```python
from build123d import *

# Parameters (mm, degrees)
SKETCH2_W                 = 130
SKETCH2_H                 = 130
BOSS_EXTRUDE1_DEPTH       = 3.2
CUT_EXTRUDE1_REACH        = 93.98
SKETCH4_R                 = 1.7
CUT_EXTRUDE2_REACH        = 93.98
SKETCH6_R                 = 1.7
CUT_EXTRUDE3_REACH        = 93.98
SKETCH8_R                 = 1.7
PRIMARY_WIRE_HOLE_REACH   = 93.98
SKETCH9_R                 = 2.25
SECONDARY_WIRE_HOLE_REACH = 93.98
SKETCH10_R                = 1.25
CUT_EXTRUDE6_REACH        = 93.98


with BuildPart() as part:
    # Sketch2 → Boss-Extrude1 (new body)
    with BuildSketch(Plane(origin=(0, 0, 0), x_dir=(1, 0, 0), z_dir=(0, 1, 0))):
        Rectangle(SKETCH2_W, SKETCH2_H)
    extrude(amount=BOSS_EXTRUDE1_DEPTH)

    # Sketch4 → Cut-Extrude1 (cut, up to next)
    with BuildSketch(Plane(origin=(0, 3.2, 0), x_dir=(1, 0, 0), z_dir=(0, 1, 0)), mode=Mode.PRIVATE) as cut_extrude1_sk1:
        with Locations(Location((-57.3, 57.3, 0), (0, 0, 270))):
            Circle(SKETCH4_R)
    cut_extrude1_tool1 = extrude(cut_extrude1_sk1.sketch, amount=-CUT_EXTRUDE1_REACH, mode=Mode.PRIVATE) & part.part
    # Sketch4 → Cut-Extrude1 (cut, up to next)
    with BuildSketch(Plane(origin=(0, 3.2, 0), x_dir=(1, 0, 0), z_dir=(0, 1, 0)), mode=Mode.PRIVATE) as cut_extrude1_sk2:
        with Locations(Location((57.3, 57.3, 0), (0, 0, 270))):
            Circle(SKETCH4_R)
    cut_extrude1_tool2 = extrude(cut_extrude1_sk2.sketch, amount=-CUT_EXTRUDE1_REACH, mode=Mode.PRIVATE) & part.part
    # Sketch4 → Cut-Extrude1 (cut, up to next)
    with BuildSketch(Plane(origin=(0, 3.2, 0), x_dir=(1, 0, 0), z_dir=(0, 1, 0)), mode=Mode.PRIVATE) as cut_extrude1_sk3:
        with Locations(Location((57.3, -57.3, 0), (0, 0, 270))):
            Circle(SKETCH4_R)
    cut_extrude1_tool3 = extrude(cut_extrude1_sk3.sketch, amount=-CUT_EXTRUDE1_REACH, mode=Mode.PRIVATE) & part.part
    # Sketch4 → Cut-Extrude1 (cut, up to next)
    with BuildSketch(Plane(origin=(0, 3.2, 0), x_dir=(1, 0, 0), z_dir=(0, 1, 0)), mode=Mode.PRIVATE) as cut_extrude1_sk4:
        with Locations(Location((-57.3, -57.3, 0), (0, 0, 270))):
            Circle(SKETCH4_R)
    cut_extrude1_tool4 = extrude(cut_extrude1_sk4.sketch, amount=-CUT_EXTRUDE1_REACH, mode=Mode.PRIVATE) & part.part
    add(cut_extrude1_tool1.solids().sort_by_distance((-57.3, 3.2, -57.3))[0], mode=Mode.SUBTRACT)
    add(cut_extrude1_tool2.solids().sort_by_distance((57.3, 3.2, -57.3))[0], mode=Mode.SUBTRACT)
    add(cut_extrude1_tool3.solids().sort_by_distance((57.3, 3.2, 57.3))[0], mode=Mode.SUBTRACT)
    add(cut_extrude1_tool4.solids().sort_by_distance((-57.3, 3.2, 57.3))[0], mode=Mode.SUBTRACT)

    # Sketch6 → Cut-Extrude2 (cut, up to next)
    with BuildSketch(Plane(origin=(0, 3.2, 0), x_dir=(1, 0, 0), z_dir=(0, 1, 0)), mode=Mode.PRIVATE) as cut_extrude2_sk1:
        with Locations(Location((-40.305086528, 40.305086528, 0), (0, 0, 270))):
            Circle(SKETCH6_R)
    cut_extrude2_tool1 = extrude(cut_extrude2_sk1.sketch, amount=-CUT_EXTRUDE2_REACH, mode=Mode.PRIVATE) & part.part
    # Sketch6 → Cut-Extrude2 (cut, up to next)
    with BuildSketch(Plane(origin=(0, 3.2, 0), x_dir=(1, 0, 0), z_dir=(0, 1, 0)), mode=Mode.PRIVATE) as cut_extrude2_sk2:
        with Locations(Location((40.305086528, 40.305086528, 0), (0, 0, 270))):
            Circle(SKETCH6_R)
    cut_extrude2_tool2 = extrude(cut_extrude2_sk2.sketch, amount=-CUT_EXTRUDE2_REACH, mode=Mode.PRIVATE) & part.part
    # Sketch6 → Cut-Extrude2 (cut, up to next)
    with BuildSketch(Plane(origin=(0, 3.2, 0), x_dir=(1, 0, 0), z_dir=(0, 1, 0)), mode=Mode.PRIVATE) as cut_extrude2_sk3:
        with Locations(Location((40.305086528, -40.305086528, 0), (0, 0, 270))):
            Circle(SKETCH6_R)
    cut_extrude2_tool3 = extrude(cut_extrude2_sk3.sketch, amount=-CUT_EXTRUDE2_REACH, mode=Mode.PRIVATE) & part.part
    # Sketch6 → Cut-Extrude2 (cut, up to next)
    with BuildSketch(Plane(origin=(0, 3.2, 0), x_dir=(1, 0, 0), z_dir=(0, 1, 0)), mode=Mode.PRIVATE) as cut_extrude2_sk4:
        with Locations(Location((-40.305086528, -40.305086528, 0), (0, 0, 270))):
            Circle(SKETCH6_R)
    cut_extrude2_tool4 = extrude(cut_extrude2_sk4.sketch, amount=-CUT_EXTRUDE2_REACH, mode=Mode.PRIVATE) & part.part
    add(cut_extrude2_tool1.solids().sort_by_distance((-40.305087, 3.2, -40.305087))[0], mode=Mode.SUBTRACT)
    add(cut_extrude2_tool2.solids().sort_by_distance((40.305087, 3.2, -40.305087))[0], mode=Mode.SUBTRACT)
    add(cut_extrude2_tool3.solids().sort_by_distance((40.305087, 3.2, 40.305087))[0], mode=Mode.SUBTRACT)
    add(cut_extrude2_tool4.solids().sort_by_distance((-40.305087, 3.2, 40.305087))[0], mode=Mode.SUBTRACT)

    # Sketch8 → Cut-Extrude3 (cut, up to next)
    with BuildSketch(Plane(origin=(0, 3.2, 0), x_dir=(1, 0, 0), z_dir=(0, 1, 0)), mode=Mode.PRIVATE) as cut_extrude3_sk1:
        with Locations(Location((0, 9.5, 0), (0, 0, 270))):
            Circle(SKETCH8_R)
    cut_extrude3_tool1 = extrude(cut_extrude3_sk1.sketch, amount=-CUT_EXTRUDE3_REACH, mode=Mode.PRIVATE) & part.part
    # Sketch8 → Cut-Extrude3 (cut, up to next)
    with BuildSketch(Plane(origin=(0, 3.2, 0), x_dir=(1, 0, 0), z_dir=(0, 1, 0)), mode=Mode.PRIVATE) as cut_extrude3_sk2:
        with Locations(Location((8.227241336, -4.75, 0), (0, 0, 270))):
            Circle(SKETCH8_R)
    cut_extrude3_tool2 = extrude(cut_extrude3_sk2.sketch, amount=-CUT_EXTRUDE3_REACH, mode=Mode.PRIVATE) & part.part
    # Sketch8 → Cut-Extrude3 (cut, up to next)
    with BuildSketch(Plane(origin=(0, 3.2, 0), x_dir=(1, 0, 0), z_dir=(0, 1, 0)), mode=Mode.PRIVATE) as cut_extrude3_sk3:
        with Locations(Location((-8.227241336, -4.75, 0), (0, 0, 270))):
            Circle(SKETCH8_R)
    cut_extrude3_tool3 = extrude(cut_extrude3_sk3.sketch, amount=-CUT_EXTRUDE3_REACH, mode=Mode.PRIVATE) & part.part
    add(cut_extrude3_tool1.solids().sort_by_distance((0, 3.2, -9.5))[0], mode=Mode.SUBTRACT)
    add(cut_extrude3_tool2.solids().sort_by_distance((8.227241, 3.2, 4.75))[0], mode=Mode.SUBTRACT)
    add(cut_extrude3_tool3.solids().sort_by_distance((-8.227241, 3.2, 4.75))[0], mode=Mode.SUBTRACT)

    # Sketch9 → Primary wire hole (cut, up to next)
    with BuildSketch(Plane(origin=(0, 3.2, 0), x_dir=(1, 0, 0), z_dir=(0, 1, 0)), mode=Mode.PRIVATE) as primary_wire_hole_sk1:
        with Locations(Location((48.790367902, 48.790367902, 0), (0, 0, 270))):
            Circle(SKETCH9_R)
    primary_wire_hole_tool1 = extrude(primary_wire_hole_sk1.sketch, amount=-PRIMARY_WIRE_HOLE_REACH, mode=Mode.PRIVATE) & part.part
    add(primary_wire_hole_tool1.solids().sort_by_distance((48.790368, 3.2, -48.790368))[0], mode=Mode.SUBTRACT)

    # Sketch10 → Secondary wire hole (cut, up to next)
    with BuildSketch(Plane(origin=(0, 3.2, 0), x_dir=(1, 0, 0), z_dir=(0, 1, 0)), mode=Mode.PRIVATE) as secondary_wire_hole_sk1:
        with Locations(Location((22.506385739, 18.885099973, 0), (0, 0, 270))):
            Circle(SKETCH10_R)
    secondary_wire_hole_tool1 = extrude(secondary_wire_hole_sk1.sketch, amount=-SECONDARY_WIRE_HOLE_REACH, mode=Mode.PRIVATE) & part.part
    add(secondary_wire_hole_tool1.solids().sort_by_distance((22.506386, 3.2, -18.8851))[0], mode=Mode.SUBTRACT)

    # Sketch11 → Cut-Extrude6 (cut, up to next)
    with BuildSketch(Plane(origin=(0, 3.2, 0), x_dir=(1, 0, 0), z_dir=(0, 1, 0)), mode=Mode.PRIVATE) as cut_extrude6_sk1:
        with BuildLine():
            Line((-34.259927979, 48.372330261), (-15.380990703, 23.319134311))
            ThreePointArc((-15.380990703, 23.319134311), (-15.725426555, 20.868345878), (-18.176214988, 21.21278173))
            Line((-18.176214988, 21.21278173), (-37.055152264, 46.26597768))
            ThreePointArc((-37.055152264, 46.26597768), (-36.710716412, 48.716766113), (-34.259927979, 48.372330261))
        make_face()
    cut_extrude6_tool1 = extrude(cut_extrude6_sk1.sketch, amount=-CUT_EXTRUDE6_REACH, mode=Mode.PRIVATE) & part.part
    # Sketch11 → Cut-Extrude6 (cut, up to next)
    with BuildSketch(Plane(origin=(0, 3.2, 0), x_dir=(1, 0, 0), z_dir=(0, 1, 0)), mode=Mode.PRIVATE) as cut_extrude6_sk2:
        with BuildLine():
            Line((-27.938203096, 52.278884913), (-13.975987518, 24.187365977))
            ThreePointArc((-13.975987518, 24.187365977), (-11.629987027, 23.399151731), (-10.841772782, 25.745152222))
            Line((-10.841772782, 25.745152222), (-24.80398836, 53.836671159))
            ThreePointArc((-24.80398836, 53.836671159), (-27.149988851, 54.624885404), (-27.938203096, 52.278884913))
        make_face()
    cut_extrude6_tool2 = extrude(cut_extrude6_sk2.sketch, amount=-CUT_EXTRUDE6_REACH, mode=Mode.PRIVATE) & part.part
    # Sketch11 → Cut-Extrude6 (cut, up to next)
    with BuildSketch(Plane(origin=(0, 3.2, 0), x_dir=(1, 0, 0), z_dir=(0, 1, 0)), mode=Mode.PRIVATE) as cut_extrude6_sk3:
        with BuildLine():
            Line((-17.87286129, 56.517128637), (-9.301329978, 26.340883824))
            ThreePointArc((-9.301329978, 26.340883824), (-7.139754963, 25.135647974), (-5.934519112, 27.297222989))
            Line((-5.934519112, 27.297222989), (-14.506050425, 57.473467801))
            ThreePointArc((-14.506050425, 57.473467801), (-16.667625439, 58.678703651), (-17.87286129, 56.517128637))
        make_face()
    cut_extrude6_tool3 = extrude(cut_extrude6_sk3.sketch, amount=-CUT_EXTRUDE6_REACH, mode=Mode.PRIVATE) & part.part
    # Sketch11 → Cut-Extrude6 (cut, up to next)
    with BuildSketch(Plane(origin=(0, 3.2, 0), x_dir=(1, 0, 0), z_dir=(0, 1, 0)), mode=Mode.PRIVATE) as cut_extrude6_sk4:
        with BuildLine():
            Line((-7.200805802, 58.836837065), (-4.310928692, 27.600231771))
            ThreePointArc((-4.310928692, 27.600231771), (-2.407156164, 26.018887355), (-0.825811748, 27.922659883))
            Line((-0.825811748, 27.922659883), (-3.715688858, 59.159265177))
            ThreePointArc((-3.715688858, 59.159265177), (-5.619461386, 60.740609593), (-7.200805802, 58.836837065))
        make_face()
    cut_extrude6_tool4 = extrude(cut_extrude6_sk4.sketch, amount=-CUT_EXTRUDE6_REACH, mode=Mode.PRIVATE) & part.part
    # Sketch11 → Cut-Extrude6 (cut, up to next)
    with BuildSketch(Plane(origin=(0, 3.2, 0), x_dir=(1, 0, 0), z_dir=(0, 1, 0)), mode=Mode.PRIVATE) as cut_extrude6_sk5:
        with BuildLine():
            Line((3.715688858, 59.159265177), (0.825811748, 27.922659883))
            ThreePointArc((0.825811748, 27.922659883), (2.407156164, 26.018887355), (4.310928692, 27.600231771))
            Line((4.310928692, 27.600231771), (7.200805802, 58.836837065))
            ThreePointArc((7.200805802, 58.836837065), (5.619461386, 60.740609593), (3.715688858, 59.159265177))
        make_face()
    cut_extrude6_tool5 = extrude(cut_extrude6_sk5.sketch, amount=-CUT_EXTRUDE6_REACH, mode=Mode.PRIVATE) & part.part
    # Sketch11 → Cut-Extrude6 (cut, up to next)
    with BuildSketch(Plane(origin=(0, 3.2, 0), x_dir=(1, 0, 0), z_dir=(0, 1, 0)), mode=Mode.PRIVATE) as cut_extrude6_sk6:
        with BuildLine():
            Line((14.506050425, 57.473467801), (5.934519112, 27.297222989))
            ThreePointArc((5.934519112, 27.297222989), (7.139754963, 25.135647974), (9.301329978, 26.340883824))
            Line((9.301329978, 26.340883824), (17.87286129, 56.517128637))
            ThreePointArc((17.87286129, 56.517128637), (16.667625439, 58.678703651), (14.506050425, 57.473467801))
        make_face()
    cut_extrude6_tool6 = extrude(cut_extrude6_sk6.sketch, amount=-CUT_EXTRUDE6_REACH, mode=Mode.PRIVATE) & part.part
    # Sketch11 → Cut-Extrude6 (cut, up to next)
    with BuildSketch(Plane(origin=(0, 3.2, 0), x_dir=(1, 0, 0), z_dir=(0, 1, 0)), mode=Mode.PRIVATE) as cut_extrude6_sk7:
        with BuildLine():
            Line((24.80398836, 53.836671159), (10.841772782, 25.745152222))
            ThreePointArc((10.841772782, 25.745152222), (11.629987027, 23.399151731), (13.975987518, 24.187365977))
            Line((13.975987518, 24.187365977), (27.938203096, 52.278884913))
            ThreePointArc((27.938203096, 52.278884913), (27.149988851, 54.624885404), (24.80398836, 53.836671159))
        make_face()
    cut_extrude6_tool7 = extrude(cut_extrude6_sk7.sketch, amount=-CUT_EXTRUDE6_REACH, mode=Mode.PRIVATE) & part.part
    # Sketch11 → Cut-Extrude6 (cut, up to next)
    with BuildSketch(Plane(origin=(0, 3.2, 0), x_dir=(1, 0, 0), z_dir=(0, 1, 0)), mode=Mode.PRIVATE) as cut_extrude6_sk8:
        with BuildLine():
            Line((34.259927979, 48.372330261), (15.380990703, 23.319134311))
            ThreePointArc((15.380990703, 23.319134311), (15.725426555, 20.868345878), (18.176214988, 21.21278173))
            Line((18.176214988, 21.21278173), (37.055152264, 46.26597768))
            ThreePointArc((37.055152264, 46.26597768), (36.710716412, 48.716766113), (34.259927979, 48.372330261))
        make_face()
    cut_extrude6_tool8 = extrude(cut_extrude6_sk8.sketch, amount=-CUT_EXTRUDE6_REACH, mode=Mode.PRIVATE) & part.part
    add(cut_extrude6_tool1.solids().sort_by_distance((-26.218071, 3.2, -34.792556))[0], mode=Mode.SUBTRACT)
    add(cut_extrude6_tool2.solids().sort_by_distance((-19.389988, 3.2, -39.012019))[0], mode=Mode.SUBTRACT)
    add(cut_extrude6_tool3.solids().sort_by_distance((-11.90369, 3.2, -41.907176))[0], mode=Mode.SUBTRACT)
    add(cut_extrude6_tool4.solids().sort_by_distance((-4.013309, 3.2, -43.379748))[0], mode=Mode.SUBTRACT)
    add(cut_extrude6_tool5.solids().sort_by_distance((4.013309, 3.2, -43.379748))[0], mode=Mode.SUBTRACT)
    add(cut_extrude6_tool6.solids().sort_by_distance((11.90369, 3.2, -41.907176))[0], mode=Mode.SUBTRACT)
    add(cut_extrude6_tool7.solids().sort_by_distance((19.389988, 3.2, -39.012019))[0], mode=Mode.SUBTRACT)
    add(cut_extrude6_tool8.solids().sort_by_distance((26.218071, 3.2, -34.792556))[0], mode=Mode.SUBTRACT)


solid = part.part
```
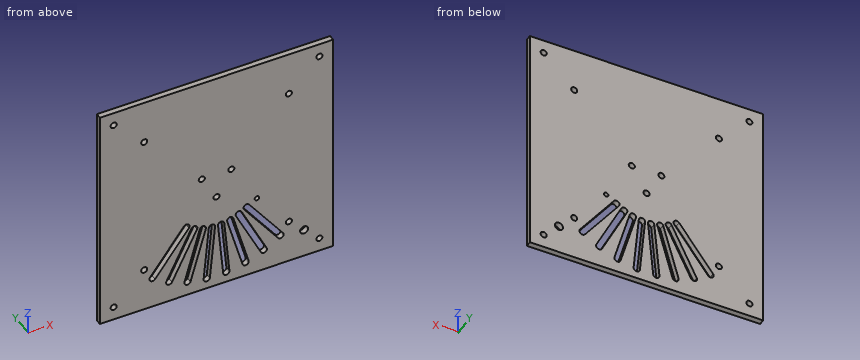
The model under review builds one solid part; all positions refer to its coordinate system, in mm. Coordinates: 2 decimals unless noted, no trailing zeros. Loops run counter-clockwise (first coordinate to the right, second up) from the corner with the lowest first, then second, coordinate; pieces in that order, holes last. Notation, with made-up numbers: (-13.5, -19) -> (-3.5, -19) arc R34 cw to (-3.5, 15) -> close; hole circle Ø10 at (32.25, 20.25). An arc over 180 degrees is marked (long way). Answer as CSV lines item,"result".
Item 1: For L1, parallel to X at y = 1.65, z = 57.3; L2, parallel to X at y = 1.05, z = 40.5; L3, parallel to Z at x = 18.5, y = 1.45, list the stretches that pass through material, from the lowest coordinate up.
Results below:
L1,"x = -65 to -59, -55.6 to 55.6, 59 to 65"
L2,"x = -65 to -41.99, -38.62 to 38.62, 41.99 to 65"
L3,"z = -65 to -41.15, -33.29 to -27.46, -21.64 to 65"
Item 2: Take a section at C-C, the plane z = 4.75. State the section outline as (x, y) points.
Results below:
outline,"(-65, 0) -> (-9.93, 0) -> (-9.93, 3.2) -> (-65, 3.2) -> close; (-6.53, 0) -> (6.53, 0) -> (6.53, 3.2) -> (-6.53, 3.2) -> close; (9.93, 0) -> (65, 0) -> (65, 3.2) -> (9.93, 3.2) -> close"
Item 3: Insertion check: pin 1 (10 mm diameter, centred on x = -28.5, z = 25.5, fed in from -Y). The pin has a flat end and moves straight along its axis. Give the tip position at first contact, or say it passes through.
Results below:
pin 1,"stops at y = 0"
Item 4: Take a section at D-D, the plane x = -31.5. State the section outline as (y, z) points.
Results below:
outline,"(0, -65) -> (3.2, -65) -> (3.2, -44.71) -> (0, -44.71) -> close; (0, -38.89) -> (3.2, -38.89) -> (3.2, 65) -> (0, 65) -> close"
Item 5: Take a section at A-A, the plane x = -57.3. State the section outline as (y, z) points.
Results below:
outline,"(0, -65) -> (3.2, -65) -> (3.2, -59) -> (0, -59) -> close; (0, -55.6) -> (3.2, -55.6) -> (3.2, 55.6) -> (0, 55.6) -> close; (0, 59) -> (3.2, 59) -> (3.2, 65) -> (0, 65) -> close"
Item 6: Take a section at B-B, the plane z = -9.5. State the section outline as (x, y) points, and give its area (3 significant figures).
Results below:
outline,"(-65, 0) -> (-1.7, 0) -> (-1.7, 3.2) -> (-65, 3.2) -> close; (1.7, 0) -> (65, 0) -> (65, 3.2) -> (1.7, 3.2) -> close"
area,"405 mm2"
